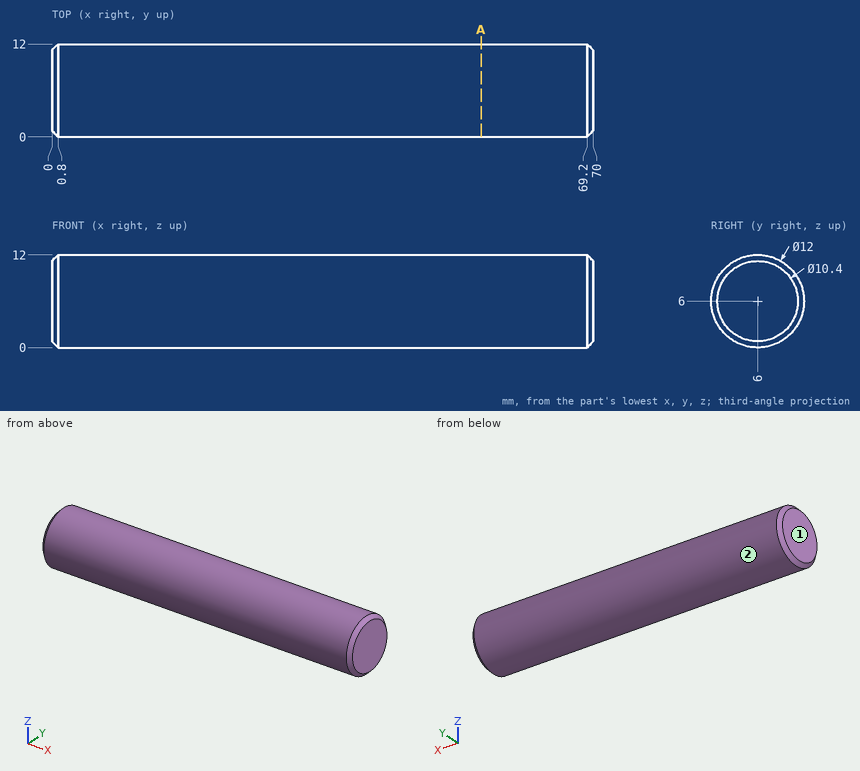
Source: three-view drawing plus pictorial views. Frame: mm from the lowest corner of the part. Coordinates: 2 decimals unless noted, no trailing zeros. Order: outer loops, then holes, each group sorted by start corner. A loop starts at its lowest first (then second) coordinate and runs counter-clockwise, first axis right, second up. Notation, with made-up numbers: M 84.25,70 L 96.25,70 A27 cw 96.25,106 Z; hole C 50.25,-0.5 d1. An arc over 180 degrees is marked long. Write each question's results on one line, items separated by ' | '. Start each with the question number.
1. Material intervals for L1, parallel to X at y = 2.5, z = 1.75; L2, parallel to X at y = 2.5, z = 1.25; L3, parallel to Z at x = 39, y = 10.25, sorted ascending.
2. Section A-A, the plane x = 55.5. Return the cut outline in (y, z).
3. Draft query along Y for the marked faces 1 and 2. Return one class per face: +Y half, -Y half, draft (parallel to the pull), parting line (faces both ways), or undercut.
4. Pin query (flat end, axial travel): pin 1 (4 mm diameter, centred on x = 22, z = 6.5, fed in from -Y); pin 2 (3 mm diameter, centred on x = 43, y = 3.5, fed in from -Z). Return the tip coordinate at first contact, or that it passes through.
Solution:
1) L1: 0.31 to 69.69 | L2: 0.7 to 69.3 | L3: 1.76 to 10.24
2) outline: C 6,6 d12
3) face 1: draft | face 2: parting line
4) pin 1: y = 0 | pin 2: z = 0.08
